Verification items for this drawing (mm, ordinates from the low corner). A direction names the side the tool comes from. Coordinates: 2 decimals unless noted, no trailing zeros. Order: outer loops, then holes, each group sorted by start corner. A loop starts at its lowest first (then second) coordinate and runs counter-clockwise, first axis right, second up. Notation, with made-up numbers: (34.25, 54) -> (70.25, 54) arc R28 ccw to (70.25, 76) -> close; hole circle Ø5 at (-39, 40). An arc over 180 degrees is marked (long way). Write item = value, one per line. Start each with the question number.
1. Thickness scan on line 1 along X through (y, z) = (3.2, 10); line 2 along X through (y, z) = (3.25, 10.5) (1 decimal); line 3 along Y through (x, z) = (6.75, 5.75). Record the ranges inside material, lowest first. Write a range as from..to.
2. Cross-section at A-A on z = 10. Give the number of separate pieces and of enclosed holes in the cut face, plus the area to 3 significant figures.
3. Go/stop test with flat-tipped pins: P1, Ø4.5, axis at x = 10, z = 10, coming from the -Y side; P2, Ø1.8, axis at x = 10, z = 15, coming from the +Y side; P3, Ø1, axis at x = 4.5, z = 12, coming from the -Y side. Record where each tip stops, or that it passes through.
4. Cross-section at C-C on y = 2.5. Record the cut outline in (x, z), plus the area to 3 significant figures.
5. Release check for a two-part mould opening along X. For the marked faces 3, 4 and 5 record: +X half, -X half, draft (parallel to the pull), parting line (faces both ways), or undercut.
6. Cross-section at D-D on z = 15.5. Record the cut outline in (x, y) (1 decimal).
7. Cross-section at B-B on x = 15. Record the cut outline in (y, z).
8. Set-up check for the marked faces 1 and 2: record each of +Z, -Z, +X, -X, +Y, -Y from which the full face is reachable in a straight line by a thin tool's end or side.
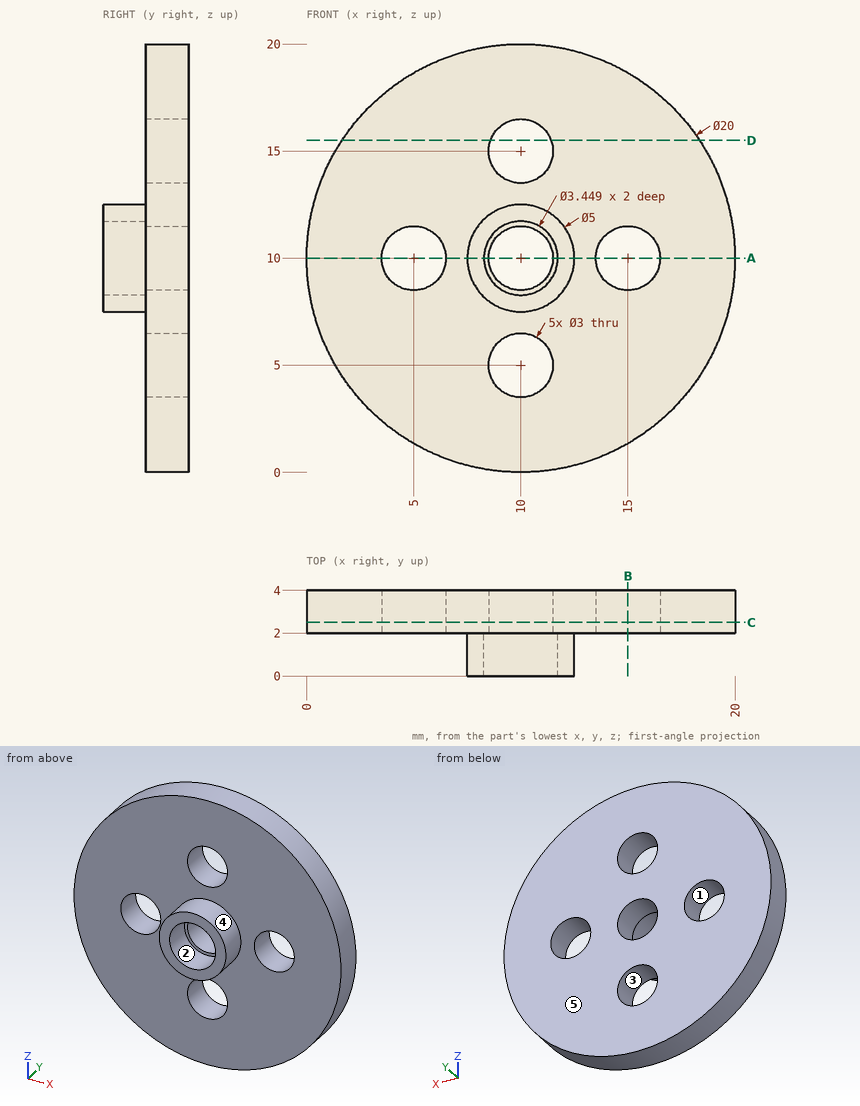
Worked out:
q1.line_1 = 0..3.5, 6.5..8.5, 11.5..13.5, 16.5..20
q1.line_2 = 0..3.6, 6.4..8.6, 11.4..13.6, 16.4..20
q1.line_3 = 2..4
q2.separate_pieces = 4
q2.enclosed_holes = 0
q2.area = 25.1 mm²
q3.P1 = 0
q3.P2 = through
q3.P3 = 2
q4.outline = circle Ø20 at (10, 10); hole circle Ø3 at (5, 10); hole circle Ø3 at (10, 5); hole circle Ø3 at (10, 10); hole circle Ø3 at (10, 15); hole circle Ø3 at (15, 10)
q4.area = 279 mm²
q5.face_3 = undercut
q5.face_4 = parting line
q5.face_5 = draft
q6.outline = (1.6, 2) -> (8.6, 2) -> (8.6, 4) -> (1.6, 4) -> close; (11.4, 2) -> (18.4, 2) -> (18.4, 4) -> (11.4, 4) -> close
q7.outline = (2, 1.34) -> (4, 1.34) -> (4, 8.5) -> (2, 8.5) -> close; (2, 11.5) -> (4, 11.5) -> (4, 18.66) -> (2, 18.66) -> close
q8.face_1 = +Y, -Y
q8.face_2 = -Y
